```python
from build123d import *

# Parameters (mm, degrees)
SKETCH_1_R      = 32.5
SKETCH_1_R_2    = 1.7
EXTRUDE_1_DEPTH = 5
SKETCH_2_R      = 55
SKETCH_2_R_2    = 3.7
EXTRUDE_2_DEPTH = 5
FILLET_2_R      = 3
FILLET_3_R      = 3


with BuildPart() as part:
    # 草图1 → 凸台-拉伸1 (new body)
    with BuildSketch(Plane.XY):
        Circle(SKETCH_1_R)
        with Locations((-13.435028843, 13.435028843)):
            Circle(SKETCH_1_R_2, mode=Mode.SUBTRACT)
        with Locations((-13.435028843, -13.435028843)):
            Circle(SKETCH_1_R_2, mode=Mode.SUBTRACT)
        with Locations((13.435028843, -13.435028843)):
            Circle(SKETCH_1_R_2, mode=Mode.SUBTRACT)
        with Locations((13.435028843, 13.435028843)):
            Circle(SKETCH_1_R_2, mode=Mode.SUBTRACT)
    extrude(amount=EXTRUDE_1_DEPTH)

    # 草图2 → 凸台-拉伸2 (add)
    with BuildSketch(Plane.XY.offset(5)):
        Circle(SKETCH_2_R)
        with Locations((13.435028843, -13.435028843)):
            Circle(SKETCH_2_R_2, mode=Mode.SUBTRACT)
        with Locations((-13.435028843, 13.435028843)):
            Circle(SKETCH_2_R_2, mode=Mode.SUBTRACT)
        with Locations((-13.435028843, -13.435028843)):
            Circle(SKETCH_2_R_2, mode=Mode.SUBTRACT)
        with Locations((13.435028843, 13.435028843)):
            Circle(SKETCH_2_R_2, mode=Mode.SUBTRACT)
    extrude(amount=EXTRUDE_2_DEPTH)

    # 圆角2
    fillet_2_edges = [part.edges().sort_by_distance(p)[0] for p in [
        (-32.5, 0, 0),
    ]]
    fillet(fillet_2_edges, radius=FILLET_2_R)

    # 圆角3
    fillet_3_edges = [part.edges().sort_by_distance(p)[0] for p in [
        (-55, 0, 5),
    ]]
    fillet(fillet_3_edges, radius=FILLET_3_R)


solid = part.part
```
Work out the finished part from the listing and answer in its coordinate system (mm). A direction names the side the tool comes from. Give positions to 0.01 mm unless a question says otherwise; leave off trailing zeros. Write each loop counter-clockwise with the first axis right and the second up, starting at its lowest first coordinate (ties: lowest second). Pieces come first, ordered by that corner, then holes. Notation, with made-up numbers: (8.5, -29) -> (41.5, -29) arc R8 ccw to (41.5, -14) -> close; hole circle Ø4 at (14.5, 39). An arc over 180 degrees is marked (long way). Write item = value, one per line.
Q1. A tool of negligible diameter and unlimited length cuts with its end or side. For faces 5 (the flat face through (0, 0, 0)), 6 (the cylindrical face through (-14.237, -17.047, 7.465)), from which of +Z, -Z, +X, -X, +Y, -Y can it reach the whole face along a straight path? Write none if from no direction.
Computed values:
face_5 = -Z, +X, -X, +Y, -Y
face_6 = +Z
Q2. For a pull along Y with two mould halves and no side action, classify faces 1 (the cylindrical face through (31, 9.76, 3.99)), 2 (the cylindrical face through (14.3, 14.9, 2.5)), 3 (the cylindrical face through (-17.13, 13.6, 7.46)), 4 (the flat face through (22.4, 23.8, 5)) as pulls with the +Y half, pulls with the -Y half, needs draft (parallel to the pull), parting line crosses it, or undercut.
Computed values:
face_1 = parting line crosses it
face_2 = undercut
face_3 = undercut
face_4 = needs draft
Q3. Flat-ended cylindrical pins translate along their axes: pin 1 Ø2 at (x, z) = (34.5, 4.5) entering from +Y; pin 2 Ø4 at (x, z) = (-2.5, 8.5) entering from +Y; pin 3 Ø3.5 at (x, y) = (12, -14) entering from +Z. Find the tip coordinate at first contact, or state that the pin passes through.
Computed values:
pin_1 = 41.26
pin_2 = 55
pin_3 = 5
Q4. Consider line 1 along X through (y, z) = (16, 8); line 2 along Z through (x, y) = (15, -34.5); line 3 along X through (y, z) = (38, 7). Determine where each line is inside the solid, lowest interval first.
Computed values:
line_1 = -52.62 to -16.1, -10.77 to 10.77, 16.1 to 52.62
line_2 = 5 to 10
line_3 = -39.52 to 39.52
Q5. Section A-A on x = 0 is taken. Determine the outline of the cut face in (y, z), and give its area (3 significant figures).
Computed values:
outline = (-55, 8) arc R3 ccw to (-52, 5) -> (-32.5, 5) -> (-32.5, 3) arc R3 ccw to (-29.5, 0) -> (29.5, 0) arc R3 ccw to (32.5, 3) -> (32.5, 5) -> (52, 5) arc R3 ccw to (55, 8) -> (55, 10) -> (-55, 10) -> close
area = 867 mm^2
